from build123d import *

# Parameters (mm, degrees)
F1_DEPTH = 76.2
F3_D     = 6.35


with BuildPart() as f1:
    # F0 (on Front) → F1 (new body)
    with BuildSketch(Plane.XZ):
        with BuildLine():
            Line((24.416897, 50.195754), (0, 62.235206))
            ThreePointArc((0, 62.235206), (-31.117603, 31.117603), (0, 0))
            Line((0, 0), (32.941068, 0))
            Line((32.941068, 0), (69.759652, 15.642613))
            Line((69.759652, 15.642613), (55.079527, 50.195754))
            Line((55.079527, 50.195754), (24.416897, 50.195754))
        make_face()
    extrude(amount=F1_DEPTH)

    # F3 (through all)
    with Locations(Plane.XZ.offset(76.2)):
        with Locations((32.941068, 29.335953), (55.079527, 29.335953), (0, 31.117603)):
            Hole(F3_D / 2)


solid = f1.part
Design review of the part built by this model. Coordinates are the model's own, in mm. A direction names the side the tool comes from. Coordinates: 2 decimals unless noted, no trailing zeros. Write each loop counter-clockwise with the first axis right and the second up, starting at its lowest first coordinate (ties: lowest second). Pieces come first, ordered by that corner, then holes. Notation, with made-up numbers: (-37.75, -17) - (-15.75, -17) arc R28 cw to (-15.75, 19) - close; hole circle Ø7 at (-33, -9). An arc over 180 degrees is marked (long way). Use one line per item in the form item = value.
Q1. Consider section A-A (y = -20.5). Write out the cut boundary in (x, z) (3 decimals).
Taken from the geometry:
outline = (0, 0) - (32.941, 0) - (69.76, 15.643) - (55.08, 50.196) - (24.417, 50.196) - (0, 62.235) arc R31.118 ccw to start; hole circle Ø6.35 at (0, 31.118); hole circle Ø6.35 at (32.941, 29.336); hole circle Ø6.35 at (55.08, 29.336)
Q2. Insertion check: pin 1 Ø4 at (x, y) = (32, -55.5) entering from +Z; pin 2 Ø8.5 at (x, z) = (55.08, 29.34) entering from +Y; pin 3 Ø5 at (x, z) = (0, 31.12) entering from -Y; pin 4 Ø2 at (y, z) = (-58, 40) entering from -X. Each pin has a flat end and moves straight along its axis. Give the tip position at first contact, or say it passes through.
Taken from the geometry:
pin_1 = 50.2
pin_2 = 0
pin_3 = through
pin_4 = -30.1
Q3. Machinability: for faces 4 (the flat face through (40, -38, 50.196)), 5 (the cylindrical face through (-31.11, -37.57, 31.8)), which of the approach directions +Z, -Z, +X, -X, +Y, -Y give a long, thin tool a straight path to every point of the face, cutting with its end or side? Answer none if there is none.
Taken from the geometry:
face_4 = +Z, +X, +Y, -Y
face_5 = -X, +Y, -Y
Q4. Consider section C-C (z = 46). Write out the cut boundary in (x, y), plus the area to 3 significant figures.
Taken from the geometry:
outline = (-27.33, -76.2) - (56.86, -76.2) - (56.86, 0) - (-27.33, 0) - close
area = 6,420 mm^2
Q5. The part is to be moulded in two halves that separate along X. For faces 1 (the cylindrical face through (33.629, -37.567, 26.236)), 2 (the flat face through (16, -38, 0)), 3 (the flat face through (51.09, -37.57, 7.71)), say which applies: +X half, -X half, draft (parallel to the pull), parting line (faces both ways), or undercut.
Taken from the geometry:
face_1 = undercut
face_2 = draft
face_3 = +X half
Q6. For probe 1 along Z at (x, y) = (0, -41); probe 2 along X at (y, z) = (-58, 29); probe 3 along X at (y, z) = (-57, 34), list the stretches that pass through material, from the lowest coordinate up.
Taken from the geometry:
probe_1 = 0 to 27.94, 34.29 to 62.24
probe_2 = -31.05 to -2.37, 2.37 to 29.78, 36.1 to 51.92, 58.24 to 64.08
probe_3 = -30.98 to -1.33, 1.33 to 61.96
Q7. Consider section B-B (x = 27). Write out the cut boundary in (y, z), plus the area to 3 significant figures.
Taken from the geometry:
outline = (-76.2, 0) - (0, 0) - (0, 50.2) - (-76.2, 50.2) - close
area = 3,820 mm^2
